```python
from build123d import *

# Parameters (mm, degrees)
F2_DEPTH = 4
F3_W     = 63.5204769373
F3_H     = 10
F3_W_2   = 10
F3_W_3   = 63.4795230627
F4_DEPTH = 20
F5_W     = 10.3620196581
F5_H     = 10
F5_W_2   = 10.2485753596
F5_W_3   = 10
F5_H_2   = 8.5477627644
F5_H_3   = 10.3687997332
F6_DEPTH = 40
F7_W     = 63.041254878
F7_H     = 61.1792467535
F8_DEPTH = 25


with BuildPart() as f2:
    # F0 (on Top) → F2 (new body)
    with BuildSketch(Plane.XY):
        with BuildLine():
            Line((-40, 119.2820323028), (-40, 69.2820323028))
            ThreePointArc((-40, 69.2820323028), (0, -80), (40, 69.2820323028))
            Line((40, 69.2820323028), (40, 119.2820323028))
            Line((40, 119.2820323028), (-40, 119.2820323028))
        make_face()
    extrude(amount=F2_DEPTH)

    # F3 (on face) → F4 (join)
    with BuildSketch(Plane.XY):
        Polygon((5, 114.8120965233), (0, 114.8120965233), (-5, 114.8120965233), (-5, 2.3505634069), (5, 2.3505634069), align=None)
        with Locations((36.7602384686, -2.6494365931)):
            Rectangle(F3_W, F3_H)
        with Locations((0, -2.6494365931)):
            Rectangle(F3_W_2, F3_H)
        with Locations((-36.7397615314, -2.6494365931)):
            Rectangle(F3_W_3, F3_H)
        Polygon((5, -65.1879034767), (5, -7.6494365931), (-5, -7.6494365931), (-5, -65.1879034767), (0, -65.1879034767), align=None)
    extrude(amount=-F4_DEPTH)

    # F5 (on face) → F6 (join)
    with BuildSketch(Plane(origin=(0, 0, -20), x_dir=(1, 0, 0), z_dir=(0, 0, -1))):
        with Locations((63.3394671082, 2.6494365931)):
            Rectangle(F5_W, F5_H)
        with Locations((-63.3552353829, 2.6494365931)):
            Rectangle(F5_W_2, F5_H)
        with Locations((0, 60.9140220945)):
            Rectangle(F5_W_3, F5_H_2)
        with Locations((0, -109.6276966567)):
            Rectangle(F5_W_3, F5_H_3)
    extrude(amount=F6_DEPTH)

    # F7 (on face) → F8 (join)
    with BuildSketch(Plane.XY.offset(4)):
        with Locations((-31.520627439, 30.5896233767)):
            Rectangle(F7_W, F7_H)
    extrude(amount=F8_DEPTH)


solid = f2.part
```
The listing builds one solid part. Answer for the finished solid, in the listing's coordinates (mm). A direction names the side the tool comes from. Give positions to 0.01 mm unless a question says otherwise; leave off trailing zeros. Order: outer loops, then holes, each group sorted by start corner. A loop starts at its lowest first (then second) coordinate and runs counter-clockwise, first axis right, second up. Notation, with made-up numbers: (89, -36) - (135, -36) arc R16 ccw to (135, -12) - close; hole circle Ø10 at (36.5, 54.25). An arc over 180 degrees is marked (long way). Use one line per item in the form item = value. Start each with the question number.
(1) A cutting plane is placed at A-A, the plane z = -43.5. Write down the section's boundary in (x, y), then the cut area to 3 significant figures.
(2) A cutting plane is placed at D-D, the plane x = -20.5. Write down the section's boundary in (y, z), then the cut area to 3 significant figures.
(3) A cutting plane is placed at C-C, the plane z = -14.5. Write down the section's boundary in (x, y), then the cut area to 3 significant figures.
(4) Consider line 1 (Y direction, x = -3.5, z = -25); line 2 (Z direction, x = 24, y = 98); line 3 (X direction, y = -47, z = -17). Determine where each line is inside the solid, lowest interval first. Write a range as from..to.
(5) Flat-ended cylindrical pins translate along their axes: pin 1 Ø5 at (x, y) = (51, 22.5) entering from +Z; pin 2 Ø3.5 at (x, y) = (-58.5, 57.5) entering from -Z; pin 3 Ø20 at (x, z) = (-35.5, 15.5) entering from -Y. Find the tip coordinate at first contact, or state that the pin passes through.
(6) The mould has two halves that part along Y. Classify faces 5 (the flat face through (5, -43, -16)), 6 (the flat face through (-44, -7.649, -16)), 7 (the flat face through (0, 104.443, -40)): released by +Y, released by -Y, zero draft, split by the parting line, or undercut.
(7) A cutting plane is placed at B-B, the plane y = 93. Write down the section's boundary in (x, z), then the cut area to 3 significant figures.
(8) For faces 1 (the flat face through (0, -56.64, -40)), 2 (the flat face through (68.52, -3, -30)), 3 (the flat face through (-68.48, -3, -30)), 4 (the flat face through (-63.041, 30, 16)), determine the directions among +Z, -Z, +X, -X, +Y, -Y from which every point of the face is accessible in a straight line to the end or side of a thin tool.
Ans:
q1.outline = (-68.48, -7.65) - (-58.23, -7.65) - (-58.23, 2.35) - (-68.48, 2.35) - close; (-5, -65.19) - (5, -65.19) - (5, -56.64) - (-5, -56.64) - close; (-5, 104.44) - (5, 104.44) - (5, 114.81) - (-5, 114.81) - close; (58.16, -7.65) - (68.52, -7.65) - (68.52, 2.35) - (58.16, 2.35) - close
q1.area = 395 mm^2
q2.outline = (-77.33, 0) - (-7.65, 0) - (-7.65, -20) - (2.35, -20) - (2.35, 0) - (119.28, 0) - (119.28, 4) - (61.18, 4) - (61.18, 29) - (0, 29) - (0, 4) - (-77.33, 4) - close
q2.area = 2,520 mm^2
q3.outline = (-68.48, -7.65) - (-5, -7.65) - (-5, -65.19) - (5, -65.19) - (5, -7.65) - (68.52, -7.65) - (68.52, 2.35) - (5, 2.35) - (5, 114.81) - (-5, 114.81) - (-5, 2.35) - (-68.48, 2.35) - close
q3.area = 3,070 mm^2
q4.line_1 = -65.19..-56.64, 104.44..114.81
q4.line_2 = 0..4
q4.line_3 = -5..5
q5.pin_1 = 4
q5.pin_2 = 4
q5.pin_3 = 0
q6.face_5 = zero draft
q6.face_6 = released by -Y
q6.face_7 = undercut
q7.outline = (-40, 0) - (-5, 0) - (-5, -20) - (5, -20) - (5, 0) - (40, 0) - (40, 4) - (-40, 4) - close
q7.area = 520 mm^2
q8.face_1 = -Z, +X, -X
q8.face_2 = -Z, +X, +Y, -Y
q8.face_3 = -Z, -X, +Y, -Y
q8.face_4 = +Z, -X, +Y, -Y
